Design review of the part built by this model. Coordinates are the model's own, in mm. Face numbers are marked on the shaded views. Give positions to 0.01 mm unless a question says otherwise; leave off trailing zeros. Order: outer loops, then holes, each group sorted by start corner. A loop starts at its lowest first (then second) coordinate and runs counter-clockwise, first axis right, second up.
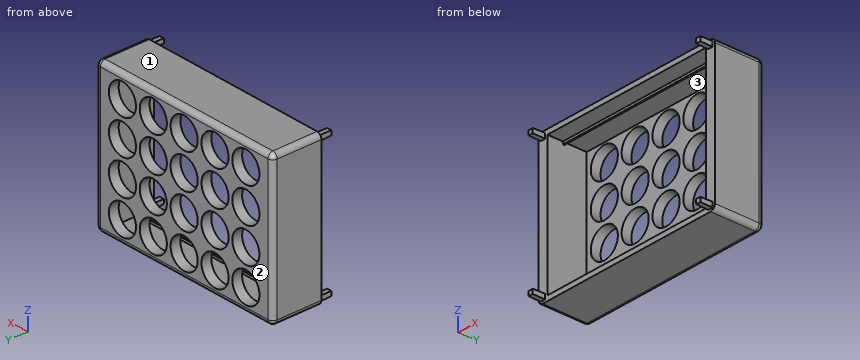
```python
from build123d import *

# Parameters (mm, degrees)
SKETCH1_W                 = 101.6
SKETCH1_H                 = 76.2
BOSS_EXTRUDE1_DEPTH       = 25.4
HOLE1_OUTLINE_R           = 7.8105
HOLE1_DEPTH               = 25.4
HOLE2_OUTLINE_R           = 7.8105
HOLE2_DEPTH               = 25.4
LPATTERN1_COUNT           = 2
LPATTERN1_PITCH           = 17.78
LPATTERN1_COPY_1_SKETCH_R = 7.8105
LPATTERN1_COPY_1_DEPTH    = 25.4
LPATTERN1_COPY_2_SKETCH_R = 7.8105
LPATTERN1_COPY_2_DEPTH    = 25.4
LPATTERN2_COPY_1_SKETCH_R = 7.8105
LPATTERN2_COPY_1_DEPTH    = 25.4
LPATTERN2_COPY_2_SKETCH_R = 7.8105
LPATTERN2_COPY_2_DEPTH    = 25.4
LPATTERN2_COPY_3_SKETCH_R = 7.8105
LPATTERN2_COPY_3_DEPTH    = 25.4
LPATTERN2_COPY_4_SKETCH_R = 7.8105
LPATTERN2_COPY_4_DEPTH    = 25.4
LPATTERN2_COPY_5_SKETCH_R = 7.8105
LPATTERN2_COPY_5_DEPTH    = 25.4
LPATTERN2_COPY_6_SKETCH_R = 7.8105
LPATTERN2_COPY_6_DEPTH    = 25.4
MIRROR2_COPY_1_SKETCH_R   = 7.8105
MIRROR2_COPY_1_DEPTH      = 25.4
MIRROR2_COPY_2_SKETCH_R   = 7.8105
MIRROR2_COPY_2_DEPTH      = 25.4
MIRROR2_COPY_3_SKETCH_R   = 7.8105
MIRROR2_COPY_3_DEPTH      = 25.4
MIRROR2_COPY_4_SKETCH_R   = 7.8105
MIRROR2_COPY_4_DEPTH      = 25.4
MIRROR2_COPY_5_SKETCH_R   = 7.8105
MIRROR2_COPY_5_DEPTH      = 25.4
MIRROR2_COPY_6_SKETCH_R   = 7.8105
MIRROR2_COPY_6_DEPTH      = 25.4
MIRROR2_COPY_7_SKETCH_R   = 7.8105
MIRROR2_COPY_7_DEPTH      = 25.4
MIRROR2_COPY_8_SKETCH_R   = 7.8105
MIRROR2_COPY_8_DEPTH      = 25.4
MIRROR2_COPY_9_SKETCH_R   = 7.8105
MIRROR2_COPY_9_DEPTH      = 25.4
MIRROR2_COPY_10_SKETCH_R  = 7.8105
MIRROR2_COPY_10_DEPTH     = 25.4
MIRROR2_COPY_11_SKETCH_R  = 7.8105
MIRROR2_COPY_11_DEPTH     = 25.4
MIRROR2_COPY_12_SKETCH_R  = 7.8105
MIRROR2_COPY_12_DEPTH     = 25.4
MIRROR2_COPY_13_SKETCH_R  = 7.8105
MIRROR2_COPY_13_DEPTH     = 25.4
MIRROR2_COPY_14_SKETCH_R  = 7.8105
MIRROR2_COPY_14_DEPTH     = 25.4
SKETCH5_W                 = 91.44
SKETCH5_H                 = 71.12
CUT_EXTRUDE1_DEPTH        = 20.32
FILLET1_R                 = 2.54
SKETCH7_W                 = 2.54
SKETCH7_H                 = 2.54
BOSS_EXTRUDE2_DEPTH       = 6.35
BOSS_EXTRUDE2_TAPER       = 1
MIRROR4_COPY_1_SKETCH_W   = 2.54
MIRROR4_COPY_1_SKETCH_H   = 2.54
MIRROR4_COPY_1_DEPTH      = 6.35
MIRROR4_COPY_1_TAPER      = 1
SKETCH9_W                 = 91.44
SKETCH9_H                 = 0.762
EXTRUDE_THIN1_DEPTH       = 1.27


# Read off the part's stored shape, not the designer's step: Hole1, Hole2
with BuildPart() as part:
    # Sketch1 → Boss-Extrude1 (new body)
    with BuildSketch(Plane(origin=(0, 0, 0), x_dir=(1, 0, 0), z_dir=(0, 1, 0))):
        Rectangle(SKETCH1_W, SKETCH1_H)
    extrude(amount=BOSS_EXTRUDE1_DEPTH)

    # Hole1 outline → Hole1 (cut)
    with BuildSketch(Plane(origin=(0, 0, 0), x_dir=(1, 0, 0), z_dir=(0, 1, 0))):
        with Locations((0, -8.89)):
            Circle(HOLE1_OUTLINE_R)
    hole1 = extrude(amount=HOLE1_DEPTH, mode=Mode.SUBTRACT)

    # Hole2 outline → Hole2 (cut)
    with BuildSketch(Plane(origin=(0, 0, 0), x_dir=(1, 0, 0), z_dir=(0, 1, 0))):
        with Locations((0, -26.67)):
            Circle(HOLE2_OUTLINE_R)
    hole2 = extrude(amount=HOLE2_DEPTH, mode=Mode.SUBTRACT)

    # Mirror1: Hole1, Hole2 across plane
    add(hole1.mirror(Plane.XY), mode=Mode.SUBTRACT)
    add(hole2.mirror(Plane.XY), mode=Mode.SUBTRACT)

    # LPattern1: Hole1, Hole2 ×2
    with Locations(*[(-i * LPATTERN1_PITCH, 0, 0) for i in range(1, LPATTERN1_COUNT)]):
        add(hole1, mode=Mode.SUBTRACT)
        add(hole2, mode=Mode.SUBTRACT)

    # LPattern1 copy 1 sketch → LPattern1 copy 1 (cut)
    with BuildSketch(Plane(origin=(-17.78, 0, 0), x_dir=(1, 0, 0), z_dir=(0, 1, 0))):
        with Locations((0, 8.89)):
            Circle(LPATTERN1_COPY_1_SKETCH_R)
    extrude(amount=LPATTERN1_COPY_1_DEPTH, mode=Mode.SUBTRACT)

    # LPattern1 copy 2 sketch → LPattern1 copy 2 (cut)
    with BuildSketch(Plane(origin=(-17.78, 0, 0), x_dir=(1, 0, 0), z_dir=(0, 1, 0))):
        with Locations((0, 26.67)):
            Circle(LPATTERN1_COPY_2_SKETCH_R)
    extrude(amount=LPATTERN1_COPY_2_DEPTH, mode=Mode.SUBTRACT)

    # LPattern2 copy 1 sketch → LPattern2 copy 1 (cut)
    with BuildSketch(Plane(origin=(-35.56, 0, 0), x_dir=(1, 0, 0), z_dir=(0, 1, 0))):
        with Locations((0, -8.89)):
            Circle(LPATTERN2_COPY_1_SKETCH_R)
    extrude(amount=LPATTERN2_COPY_1_DEPTH, mode=Mode.SUBTRACT)

    # LPattern2 copy 2 sketch → LPattern2 copy 2 (cut)
    with BuildSketch(Plane(origin=(-35.56, 0, 0), x_dir=(1, 0, 0), z_dir=(0, 1, 0))):
        with Locations((0, -26.67)):
            Circle(LPATTERN2_COPY_2_SKETCH_R)
    extrude(amount=LPATTERN2_COPY_2_DEPTH, mode=Mode.SUBTRACT)

    # LPattern2 copy 3 sketch → LPattern2 copy 3 (cut)
    with BuildSketch(Plane(origin=(-35.56, 0, 0), x_dir=(1, 0, 0), z_dir=(0, 1, 0))):
        with Locations((0, 8.89)):
            Circle(LPATTERN2_COPY_3_SKETCH_R)
    extrude(amount=LPATTERN2_COPY_3_DEPTH, mode=Mode.SUBTRACT)

    # LPattern2 copy 4 sketch → LPattern2 copy 4 (cut)
    with BuildSketch(Plane(origin=(-35.56, 0, 0), x_dir=(1, 0, 0), z_dir=(0, 1, 0))):
        with Locations((0, 26.67)):
            Circle(LPATTERN2_COPY_4_SKETCH_R)
    extrude(amount=LPATTERN2_COPY_4_DEPTH, mode=Mode.SUBTRACT)

    # LPattern2 copy 5 sketch → LPattern2 copy 5 (cut)
    with BuildSketch(Plane(origin=(-17.78, 0, 0), x_dir=(1, 0, 0), z_dir=(0, 1, 0))):
        with Locations((0, -8.89)):
            Circle(LPATTERN2_COPY_5_SKETCH_R)
    extrude(amount=LPATTERN2_COPY_5_DEPTH, mode=Mode.SUBTRACT)

    # LPattern2 copy 6 sketch → LPattern2 copy 6 (cut)
    with BuildSketch(Plane(origin=(-17.78, 0, 0), x_dir=(1, 0, 0), z_dir=(0, 1, 0))):
        with Locations((0, -26.67)):
            Circle(LPATTERN2_COPY_6_SKETCH_R)
    extrude(amount=LPATTERN2_COPY_6_DEPTH, mode=Mode.SUBTRACT)

    # Mirror2 copy 1 sketch → Mirror2 copy 1 (cut)
    with BuildSketch(Plane(origin=(17.78, 0, 0), x_dir=(-1, 0, 0), z_dir=(0, 1, 0))):
        with Locations((0, 8.89)):
            Circle(MIRROR2_COPY_1_SKETCH_R)
    extrude(amount=MIRROR2_COPY_1_DEPTH, mode=Mode.SUBTRACT)

    # Mirror2 copy 2 sketch → Mirror2 copy 2 (cut)
    with BuildSketch(Plane(origin=(17.78, 0, 0), x_dir=(-1, 0, 0), z_dir=(0, 1, 0))):
        with Locations((0, 26.67)):
            Circle(MIRROR2_COPY_2_SKETCH_R)
    extrude(amount=MIRROR2_COPY_2_DEPTH, mode=Mode.SUBTRACT)

    # Mirror2 copy 3 sketch → Mirror2 copy 3 (cut)
    with BuildSketch(Plane(origin=(17.78, 0, 0), x_dir=(-1, 0, 0), z_dir=(0, 1, 0))):
        with Locations((0, -8.89)):
            Circle(MIRROR2_COPY_3_SKETCH_R)
    extrude(amount=MIRROR2_COPY_3_DEPTH, mode=Mode.SUBTRACT)

    # Mirror2 copy 4 sketch → Mirror2 copy 4 (cut)
    with BuildSketch(Plane(origin=(17.78, 0, 0), x_dir=(-1, 0, 0), z_dir=(0, 1, 0))):
        with Locations((0, -26.67)):
            Circle(MIRROR2_COPY_4_SKETCH_R)
    extrude(amount=MIRROR2_COPY_4_DEPTH, mode=Mode.SUBTRACT)

    # Mirror2 copy 5 sketch → Mirror2 copy 5 (cut)
    with BuildSketch(Plane(origin=(0, 0, 0), x_dir=(-1, 0, 0), z_dir=(0, 1, 0))):
        with Locations((0, 8.89)):
            Circle(MIRROR2_COPY_5_SKETCH_R)
    extrude(amount=MIRROR2_COPY_5_DEPTH, mode=Mode.SUBTRACT)

    # Mirror2 copy 6 sketch → Mirror2 copy 6 (cut)
    with BuildSketch(Plane(origin=(0, 0, 0), x_dir=(-1, 0, 0), z_dir=(0, 1, 0))):
        with Locations((0, 26.67)):
            Circle(MIRROR2_COPY_6_SKETCH_R)
    extrude(amount=MIRROR2_COPY_6_DEPTH, mode=Mode.SUBTRACT)

    # Mirror2 copy 7 sketch → Mirror2 copy 7 (cut)
    with BuildSketch(Plane(origin=(35.56, 0, 0), x_dir=(-1, 0, 0), z_dir=(0, 1, 0))):
        with Locations((0, 8.89)):
            Circle(MIRROR2_COPY_7_SKETCH_R)
    extrude(amount=MIRROR2_COPY_7_DEPTH, mode=Mode.SUBTRACT)

    # Mirror2 copy 8 sketch → Mirror2 copy 8 (cut)
    with BuildSketch(Plane(origin=(35.56, 0, 0), x_dir=(-1, 0, 0), z_dir=(0, 1, 0))):
        with Locations((0, 26.67)):
            Circle(MIRROR2_COPY_8_SKETCH_R)
    extrude(amount=MIRROR2_COPY_8_DEPTH, mode=Mode.SUBTRACT)

    # Mirror2 copy 9 sketch → Mirror2 copy 9 (cut)
    with BuildSketch(Plane(origin=(35.56, 0, 0), x_dir=(-1, 0, 0), z_dir=(0, 1, 0))):
        with Locations((0, -8.89)):
            Circle(MIRROR2_COPY_9_SKETCH_R)
    extrude(amount=MIRROR2_COPY_9_DEPTH, mode=Mode.SUBTRACT)

    # Mirror2 copy 10 sketch → Mirror2 copy 10 (cut)
    with BuildSketch(Plane(origin=(35.56, 0, 0), x_dir=(-1, 0, 0), z_dir=(0, 1, 0))):
        with Locations((0, -26.67)):
            Circle(MIRROR2_COPY_10_SKETCH_R)
    extrude(amount=MIRROR2_COPY_10_DEPTH, mode=Mode.SUBTRACT)

    # Mirror2 copy 11 sketch → Mirror2 copy 11 (cut)
    with BuildSketch(Plane(origin=(17.78, 0, 0), x_dir=(-1, 0, 0), z_dir=(0, 1, 0))):
        with Locations((0, 8.89)):
            Circle(MIRROR2_COPY_11_SKETCH_R)
    extrude(amount=MIRROR2_COPY_11_DEPTH, mode=Mode.SUBTRACT)

    # Mirror2 copy 12 sketch → Mirror2 copy 12 (cut)
    with BuildSketch(Plane(origin=(17.78, 0, 0), x_dir=(-1, 0, 0), z_dir=(0, 1, 0))):
        with Locations((0, 26.67)):
            Circle(MIRROR2_COPY_12_SKETCH_R)
    extrude(amount=MIRROR2_COPY_12_DEPTH, mode=Mode.SUBTRACT)

    # Mirror2 copy 13 sketch → Mirror2 copy 13 (cut)
    with BuildSketch(Plane(origin=(0, 0, 0), x_dir=(-1, 0, 0), z_dir=(0, 1, 0))):
        with Locations((0, 8.89)):
            Circle(MIRROR2_COPY_13_SKETCH_R)
    extrude(amount=MIRROR2_COPY_13_DEPTH, mode=Mode.SUBTRACT)

    # Mirror2 copy 14 sketch → Mirror2 copy 14 (cut)
    with BuildSketch(Plane(origin=(0, 0, 0), x_dir=(-1, 0, 0), z_dir=(0, 1, 0))):
        with Locations((0, 26.67)):
            Circle(MIRROR2_COPY_14_SKETCH_R)
    extrude(amount=MIRROR2_COPY_14_DEPTH, mode=Mode.SUBTRACT)

    # Sketch5 → Cut-Extrude1 (cut)
    with BuildSketch(Plane.XZ):
        Rectangle(SKETCH5_W, SKETCH5_H)
    extrude(amount=-CUT_EXTRUDE1_DEPTH, mode=Mode.SUBTRACT)

    # Fillet1
    fillet1_edges = [part.edges().sort_by_distance(p)[0] for p in [
        (-50.8, 25.4, 0),
        (0, 25.4, 38.1),
        (50.8, 25.4, 0),
        (50.8, 12.7, 38.1),
        (-50.8, 12.7, 38.1),
        (-50.8, 12.7, -38.1),
        (50.8, 12.7, -38.1),
        (0, 25.4, -38.1),
    ]]
    fillet(fillet1_edges, radius=FILLET1_R)

    # Sketch7 → Boss-Extrude2 (add)
    with BuildSketch(Plane(origin=(0, 0, 0), x_dir=(-1, 0, 0), z_dir=(0, -1, 0))):
        with Locations((48.26, -35.56)):
            Rectangle(SKETCH7_W, SKETCH7_H)
    boss_extrude2 = extrude(amount=BOSS_EXTRUDE2_DEPTH, taper=BOSS_EXTRUDE2_TAPER)

    # Mirror3: Boss-Extrude2 across plane
    add(boss_extrude2.mirror(Plane(origin=(0, 0, 0), x_dir=(0, 0, 1), z_dir=(1, 0, 0))))

    # Mirror4: Boss-Extrude2 across plane
    add(boss_extrude2.mirror(Plane.XY))

    # Mirror4 copy 1 sketch → Mirror4 copy 1 (add)
    with BuildSketch(Plane.XZ):
        with Locations((48.26, -35.56)):
            Rectangle(MIRROR4_COPY_1_SKETCH_W, MIRROR4_COPY_1_SKETCH_H)
    extrude(amount=MIRROR4_COPY_1_DEPTH, taper=MIRROR4_COPY_1_TAPER)

    # Sketch9 → Extrude-Thin1 (add)
    with BuildSketch(Plane.XY.offset(-35.56)):
        with Locations((0, 8.382)):
            Rectangle(SKETCH9_W, SKETCH9_H)
    extrude_thin1 = extrude(amount=EXTRUDE_THIN1_DEPTH)

    # Mirror5: Extrude-Thin1 across plane
    add(extrude_thin1.mirror(Plane.XY))


solid = part.part
```
1. For line 1 along Z through (x, y) = (35.56, 21.6); line 2 along X through (y, z) = (19, 22.5); line 3 along Z through (x, y) = (0.5, 11), list the stretches that pass through material, from the lowest coordinate up.
Recorded:
line 1: z = -38.1 to -34.48, -18.86 to -16.7, -1.08 to 1.08, 16.7 to 18.86, 34.48 to 38.1
line 2: x = -50.8 to -45.72, 45.72 to 50.8
line 3: z = -38.1 to -35.56, 35.56 to 38.1
2. Draft analysis for pull direction Y (two halves, no side actions). For the marked faces 1, 2 and 3, state which applies: pulls with the +Y half, pulls with the -Y half, needs draft (parallel to the pull), parting line crosses it, or undercut.
Recorded:
face 1: needs draft
face 2: pulls with the +Y half
face 3: undercut
3. Take a section at C-C (y = 18.5). State the section outline as (x, z) points.
Recorded:
outline: (-50.8, -35.56) arc R2.54 ccw to (-48.26, -38.1) - (48.26, -38.1) arc R2.54 ccw to (50.8, -35.56) - (50.8, 35.56) arc R2.54 ccw to (48.26, 38.1) - (-48.26, 38.1) arc R2.54 ccw to (-50.8, 35.56) - close; hole (-45.72, -35.56) - (45.72, -35.56) - (45.72, 35.56) - (-45.72, 35.56) - close
4. For pin 1 (23 mm diameter, centred on x = 22.5, z = 13, fed in from -Y); pin 2 (25 mm diameter, centred on x = -35.56, z = 8.89, fed in from -Y), all flat-tipped, find the tip position at first contact; note any pin that passes through.
Recorded:
pin 1: stops at y = 20.32
pin 2: stops at y = 0
5. Take a section at A-A (z = -26.67). State how many separate pieces and enclosed holes the cut face has, then the cut area to 3 significant figures.
Recorded:
separate pieces: 6
enclosed holes: 0
area: 323 mm2
